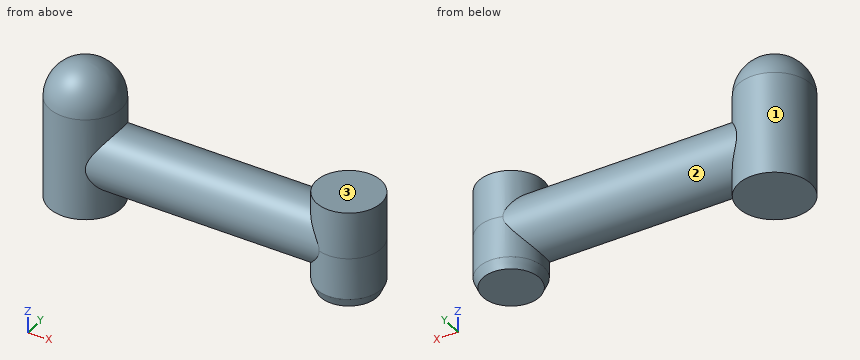
from build123d import *

# Parameters (mm, degrees)
SKETCH1_R                = 60
BOSS_EXTRUDE1_DEPTH      = 230.5
FILLET1_R                = 60
SKETCH2_R                = 51
BOSS_EXTRUDE2_DEPTH      = 438.15
SKETCH3_R                = 53.975
BOSS_EXTRUDE3_DEPTH      = 78
BOSS_EXTRUDE3_DEPTH_BACK = 85.5
CHAMFER1_SIZE            = 7
CHAMFER1_SIZE2           = 16


with BuildPart() as part:
    # Sketch1 → Boss-Extrude1 (new body)
    with BuildSketch(Plane.XY):
        Circle(SKETCH1_R)
    extrude(amount=BOSS_EXTRUDE1_DEPTH)

    # Fillet1
    fillet1_edges = [part.edges().sort_by_distance(p)[0] for p in [
        (-60, 0, 230.5),
    ]]
    fillet(fillet1_edges, radius=FILLET1_R)

    # Sketch2 → Boss-Extrude2 (add)
    with BuildSketch(Plane(origin=(0, 0, 0), x_dir=(0, 0, -1), z_dir=(1, 0, 0))):
        with Locations((-85.5, 0)):
            Circle(SKETCH2_R)
    extrude(amount=BOSS_EXTRUDE2_DEPTH)

    # Sketch3 → Boss-Extrude3 (add, two sides)
    with BuildSketch(Plane.XY.offset(85.5)) as boss_extrude3_sk:
        with Locations((438.15, 0)):
            Circle(SKETCH3_R)
    extrude(amount=BOSS_EXTRUDE3_DEPTH)
    extrude(boss_extrude3_sk.sketch, amount=-BOSS_EXTRUDE3_DEPTH_BACK)

    # Chamfer1
    chamfer1_edges = [part.edges().sort_by_distance(p)[0] for p in [
        (384.175, 0, 0),
    ]]
    chamfer1_side = [part.faces().sort_by_distance(p)[0] for p in [
        (438.15, 0, 0),
    ]]
    chamfer(chamfer1_edges, length=CHAMFER1_SIZE, length2=CHAMFER1_SIZE2, reference=chamfer1_side[0])


solid = part.part
Work out the finished part from the listing and answer in its coordinate system (mm). Face numbers are marked on the shaded views. Coordinates: 2 decimals unless noted, no trailing zeros. Order: outer loops, then holes, each group sorted by start corner. A loop starts at its lowest first (then second) coordinate and runs counter-clockwise, first axis right, second up. Notation, with made-up numbers: (-3, 39.25) - (43, 39.25) arc R16 cw to (43, 67.25) - close; hole circle Ø9 at (35.5, -36.5). An arc over 180 degrees is marked (long way). Put each result on its own line as item: value. Start each with the question number.
1) Flat-ended cylindrical pins translate along their axes: pin 1 (3 mm diameter, centred on y = -24.5, z = 191, fed in from -X); pin 2 (1 mm diameter, centred on y = -1, z = 128, fed in from +X); pin 3 (4 mm diameter, centred on y = 37, z = 141, fed in from +X). Find the tip coordinate at first contact, or state that the pin passes through.
2) Find section A-A (y = 0). Give the vertices of the cut face in (x, z) (3 decimals).
3) Find section B-B (x = 0). Give the vertices of the cut face in (y, z), plus the area to 3 significant figures.
4) Find section C-C (x = 133). Give the vertices of the cut face in (y, z), plus the area to 3 significant figures.
5) Find the intervals of material crossed by line 1 (X direction, y = 18, z = 22.5); line 2 (Z direction, x = 418.5, y = -13.5); line 3 (X direction, y = 10, z = 9.5), in increasing order. Write a range as from..to.
6) For a pull along X with two mould halves and no side action, classify the marked faces 1, 2 and 3 as released by +X, released by -X, zero draft, split by the parting line, or undercut.
Results list:
1. pin 1: stops at x = -51.7
1. pin 2: stops at x = 492.12
1. pin 3: stops at x = 479.24
2. outline: (-60, 0) - (60, 0) - (60, 34.5) - (384.175, 34.5) - (384.175, 16) - (391.175, 0) - (485.125, 0) - (492.125, 16) - (492.125, 163.5) - (384.175, 163.5) - (384.175, 136.5) - (60, 136.5) - (60, 170.5) arc R60 ccw to (-60, 170.5) - close
3. outline: (-60, 0) - (60, 0) - (60, 170.5) arc R60 ccw to (-60, 170.5) - close
3. area: 26,100 mm^2
4. outline: circle Ø102 at (0, 85.5)
4. area: 8,170 mm^2
5. line 1: x = -57.24..57.24, 387.26..489.04
5. line 2: z = 0..163.5
5. line 3: x = -59.16..59.16, 388.01..488.29
6. face 1: undercut
6. face 2: undercut
6. face 3: zero draft
